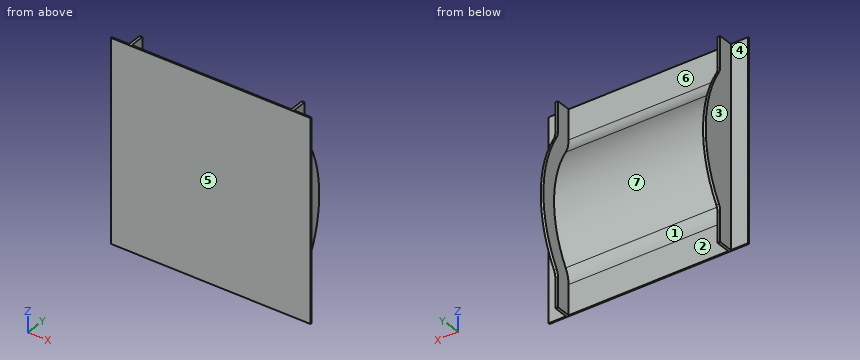
from build123d import *

# Parameters (mm, degrees)
SKETCH2_W           = 1500
SKETCH2_H           = 1500
BOSS_EXTRUDE1_DEPTH = 10
BOSS_EXTRUDE3_DEPTH = 1240
BOSS_EXTRUDE4_DEPTH = 20


with BuildPart() as part:
    # Sketch2 → Boss-Extrude1 (new body)
    with BuildSketch(Plane(origin=(0, 0, 0), x_dir=(1, 0, 0), z_dir=(0, 1, 0))):
        Rectangle(SKETCH2_W, SKETCH2_H)
    extrude(amount=BOSS_EXTRUDE1_DEPTH)

    # Sketch4 → Boss-Extrude3 (add)
    with BuildSketch(Plane.ZY.offset(620)):
        with BuildLine():
            ThreePointArc((-421.426148374, 40.000001079), (-472.010430907, 17.646159664), (-526.782687643, 10))
            Line((-526.782687643, 10), (-466.368952654, 10))
            ThreePointArc((-466.368952654, 10), (-444.150915082, 25.379564333), (-421.426148373, 40.000001079))
        make_face()
        with BuildLine():
            ThreePointArc((-421.426148373, 40.000001079), (-444.150915082, 25.379564333), (-466.368952654, 10))
            Line((-466.368952654, 10), (466.368952654, 10))
            ThreePointArc((466.368952654, 10), (444.150917669, 25.379562606), (421.426153659, 39.999997803))
            ThreePointArc((421.426153659, 39.999997803), (3.109e-06, 160), (-421.426148373, 40.000001079))
        make_face()
        with BuildLine():
            ThreePointArc((421.426153659, 39.999997803), (444.150917669, 25.379562606), (466.368952654, 10))
            Line((466.368952654, 10), (526.782687643, 10))
            ThreePointArc((526.782687643, 10), (472.010433898, 17.646158812), (421.426153659, 39.999997803))
        make_face()
    extrude(amount=-BOSS_EXTRUDE3_DEPTH)

    # Sketch5 → Boss-Extrude4 (add)
    with BuildSketch(Plane.ZY.offset(620)):
        with BuildLine():
            Line((-750, 120), (-750, 10))
            Line((-750, 10), (-526.782687643, 10))
            ThreePointArc((-526.782687643, 10), (-472.010431892, 17.646159383), (-421.426150114, 40))
            ThreePointArc((-421.426150114, 40), (-337.988327134, 85.095780378), (-249.799919936, 120))
            Line((-249.799919936, 120), (-526.782687643, 120))
            Line((-526.782687643, 120), (-750, 120))
        make_face()
        with BuildLine():
            ThreePointArc((-479.372245755, 133.5), (-502.135172555, 123.440771722), (-526.782687643, 120))
            Line((-526.782687643, 120), (-249.799919936, 120))
            ThreePointArc((-249.799919936, 120), (0, 160), (249.799919936, 120))
            Line((249.799919936, 120), (526.782687643, 120))
            ThreePointArc((526.782687643, 120), (502.135172555, 123.440771722), (479.372245755, 133.5))
            ThreePointArc((479.372245755, 133.5), (0, 270), (-479.372245755, 133.5))
        make_face()
        with BuildLine():
            ThreePointArc((421.426150114, 40), (472.010431892, 17.646159383), (526.782687643, 10))
            Line((526.782687643, 10), (750, 10))
            Line((750, 10), (750, 120))
            Line((750, 120), (526.782687643, 120))
            Line((526.782687643, 120), (249.799919936, 120))
            ThreePointArc((249.799919936, 120), (337.988327134, 85.095780378), (421.426150114, 40))
        make_face()
    boss_extrude4 = extrude(amount=-BOSS_EXTRUDE4_DEPTH)

    # Mirror1: Boss-Extrude4 across plane
    add(boss_extrude4.mirror(Plane(origin=(0, 0, 0), x_dir=(0, 0, 1), z_dir=(1, 0, 0))))


solid = part.part
Work out the finished part from the listing and answer in its coordinate system (mm). Face numbers are marked on the shaded views. A direction names the side the tool comes from. Coordinates: 2 decimals unless noted, no trailing zeros. Write each loop counter-clockwise with the first axis right and the second up, starting at its lowest first coordinate (ties: lowest second). Pieces come first, ordered by that corner, then holes.
1. Consider line 1 along X through (y, z) = (141.5, 415.5); line 2 along Y through (x, z) = (-448.5, -576); line 3 along X through (y, z) = (15.5, -438). Determine where each line is inside the solid, lowest interval first.
Results list:
line 1: x = -620 to -600, 600 to 620
line 2: y = 0 to 10
line 3: x = -620 to 620
2. The part is cut by section A-A, the plane y = 245.5. Write down the section's boundary in (x, z), and give its area (3 significant figures).
Results list:
outline: (-620, -209.74) - (-600, -209.74) - (-600, 209.74) - (-620, 209.74) - close; (600, -209.74) - (620, -209.74) - (620, 209.74) - (600, 209.74) - close
area: 16,800 mm2
3. Flat-ended cylindrical pins translate along their axes: pin 1 (8 mm diameter, centred on x = 437, z = 396, fed in from -Y); pin 2 (3 mm diameter, centred on x = -221.5, z = -247, fed in from +Y); pin 3 (4 mm diameter, centred on x = 481, z = 404.5, fed in from +Y); pin 4 (16 mm diameter, centred on x = -609, z = -595.5, fed in from +Y). Find the tip coordinate at first contact, or state that the pin passes through.
Results list:
pin 1: stops at y = 0
pin 2: stops at y = 121.4
pin 3: stops at y = 51.37
pin 4: stops at y = 120
4. The part is cut by section D-D, the plane y = 82.5. Write down the section's boundary in (x, z), and give its area (3 significant figures).
Results list:
outline: (-620, -750) - (-600, -750) - (-600, -343.5) - (600, -343.5) - (600, -750) - (620, -750) - (620, 750) - (600, 750) - (600, 343.5) - (-600, 343.5) - (-600, 750) - (-620, 750) - close
area: 884,000 mm2
5. The part is cut by section B-B, the plane x = -364. Write down the section's boundary in (y, z).
Results list:
outline: (0, -750) - (10, -750) - (10, -526.78) arc R200 cw to (40, -421.43) arc R800 ccw to (40, 421.43) arc R200 cw to (10, 526.78) - (10, 750) - (0, 750) - close
6. For a pull along X with two mould halves and no side action, classify the marked faces 1, 2, 3 and 4 as +X half, -X half, draft (parallel to the pull), parting line (faces both ways), or undercut.
Results list:
face 1: undercut
face 2: undercut
face 3: -X half
face 4: draft
7. The part is cut by section C-C, the plane z = 643.5. Write down the section's boundary in (x, y).
Results list:
outline: (-750, 0) - (750, 0) - (750, 10) - (620, 10) - (620, 120) - (600, 120) - (600, 10) - (-600, 10) - (-600, 120) - (-620, 120) - (-620, 10) - (-750, 10) - close
8. For the marked faces 5, 6 and 7, determine the directions among +Z, -Z, +X, -X, +Y, -Y from which every point of the face is accessible in a straight line to the end or side of a thin tool.
Results list:
face 5: +Z, -Z, +X, -X, -Y
face 6: +Z, +Y
face 7: +Y
